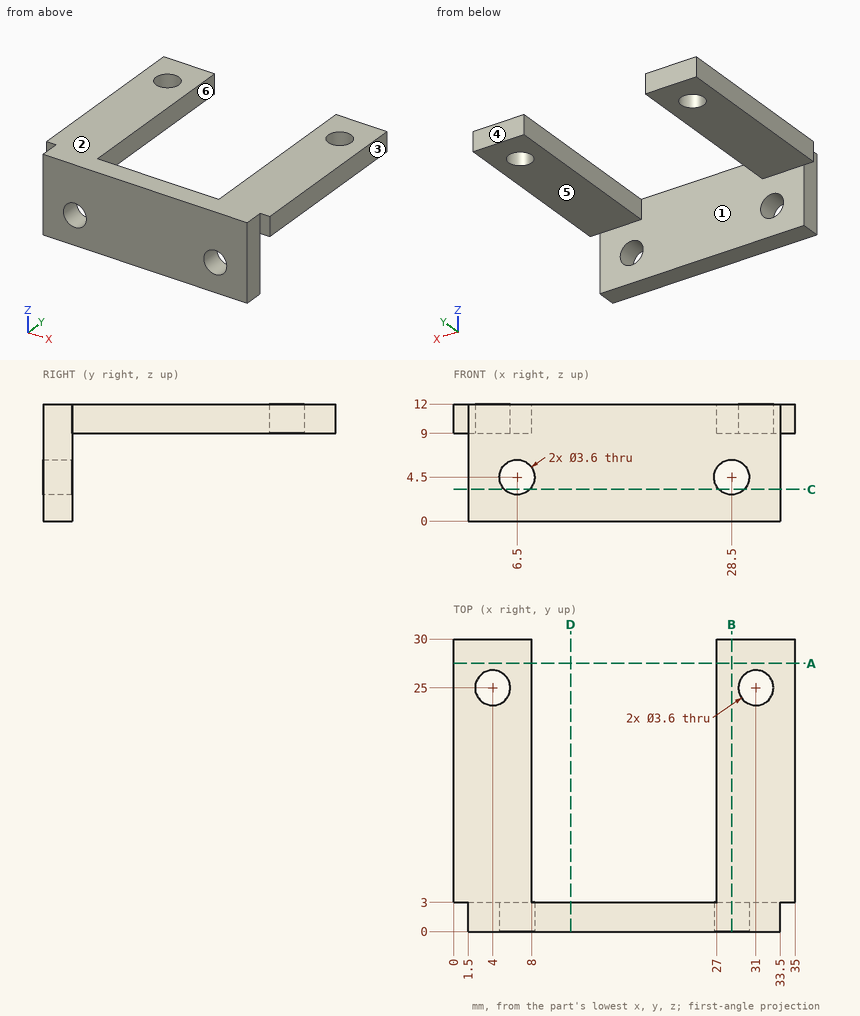
Source: three-view drawing plus pictorial views. Frame: mm from the lowest corner of the part. A direction names the side the tool comes from. Coordinates: 2 decimals unless noted, no trailing zeros. Order: outer loops, then holes, each group sorted by start corner. A loop starts at its lowest first (then second) coordinate and runs counter-clockwise, first axis right, second up.
1) Section D-D (x = 12). Return loops of the section in (y, z), then the cut area to 3 significant figures.
Result sheet:
outline: (0, 0) - (3, 0) - (3, 12) - (0, 12) - close
area: 36.0 mm2
2) Set-up query: the marked faces 4, 5 and 6. Return all of +Z, -Z, +X, -X, +Y, -Y with unobstructed straight access to the full face (end or side cutting, diameter ignored); none if empty.
Result sheet:
face 4: +Z, -Z, +X, -X, +Y
face 5: -Z, +X, -X, +Y
face 6: +Z, -Z, +Y
3) Draft query along X for the marked faces 1, 2 and 3. Return one class per face: released by +X, released by -X, zero draft, split by the parting line, or undercut.
Result sheet:
face 1: undercut
face 2: zero draft
face 3: released by +X
4) First-contact query: P1, Ø9, axis at x = 30, y = 18, coming from the -Z side; P2, Ø3, axis at x = 17.5, z = 3, coming from the +Y side; P3, Ø0.9, axis at y = 1, z = 4.5, coming from the +X side. Flat tips, straight axial feed; report the tip coordinate or a pass-through.
Result sheet:
P1: stops at z = 9
P2: stops at y = 3
P3: stops at x = 33.5
5) Section C-C (z = 3.25). Return loops of the section in (x, y).
Result sheet:
outline: (1.5, 0) - (5.2, 0) - (5.2, 3) - (1.5, 3) - close; (7.8, 0) - (27.2, 0) - (27.2, 3) - (7.8, 3) - close; (29.8, 0) - (33.5, 0) - (33.5, 3) - (29.8, 3) - close
6) Section A-A (y = 27.5). Return loops of the section in (x, z).
Result sheet:
outline: (0, 9) - (8, 9) - (8, 12) - (0, 12) - close; (27, 9) - (35, 9) - (35, 12) - (27, 12) - close
7) Section B-B (x = 28.5). Return loops of the section in (y, z).
Result sheet:
outline: (0, 0) - (3, 0) - (3, 2.7) - (0, 2.7) - close; (0, 6.3) - (3, 6.3) - (3, 9) - (30, 9) - (30, 12) - (0, 12) - close
8) Ray query, probe 1 along X at (y, z) = (1.6, 4.5); probe 2 along X at (y, z) = (12, 10); probe 3 along Y at (x, z) = (31, 11.3). Return the intervals inside material, ascending.
Result sheet:
probe 1: x = 1.5 to 4.7, 8.3 to 26.7, 30.3 to 33.5
probe 2: x = 0 to 8, 27 to 35
probe 3: y = 0 to 23.2, 26.8 to 30
